Here's how the part is built. I have some questions about the finished solid (model axes, mm). Round coordinates to 2 decimals unless told otherwise and drop trailing zeros. Loops run counter-clockwise (first coordinate to the right, second up) from the corner with the lowest first, then second, coordinate; pieces in that order, holes last. Notation, with made-up numbers: (11, 75) - (58, 75) arc R18 cw to (58, 93) - close; hole circle Ø11 at (43, 5). An arc over 180 degrees is marked (long way). Answer as a JSON object with one key per item and string values. Group by question number.
1) Will these pins go through, and if not, where does the flat tip stop? P1, Ø6, axis at y = 5.5, z = 93.5, coming from the -X side; P2, Ø13, axis at x = 12, z = 63.5, coming from the +Y side; P3, Ø9.5, axis at y = 489.5, z = 82.5, coming from the +X side.
2) If I drill on line 1 along X through (y, z) = (73, 13.5), over which ranges is the centre line in solid material (lowest first)? Write a range as [from, to].
3) I want a section at C-C, the plane z = 46.5. Please give me the cut outline in (x, y), then the cut area to 3 significant figures.
4) I want a section at A-A, the plane y = 259.5. Please give me the cut outline in (x, z).
5) I want a section at B-B, the plane x = 310. Please give me the cut outline in (y, z).
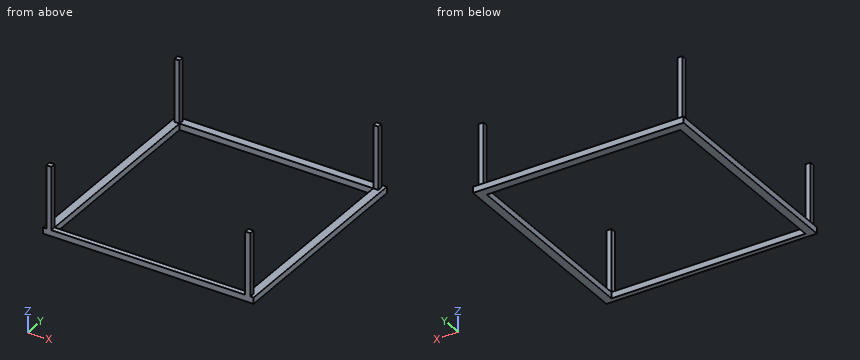
from build123d import *

# Parameters (mm, degrees)
SKETCH1_W           = 503
SKETCH1_H           = 503
SKETCH1_W_2         = 463
SKETCH1_H_2         = 471
BOSS_EXTRUDE1_DEPTH = 15
SKETCH2_W           = 12
SKETCH2_H           = 12
BOSS_EXTRUDE2_DEPTH = 200
SKETCH3_W           = 487
SKETCH3_H           = 495
CUT_EXTRUDE1_DEPTH  = 50


with BuildPart() as part:
    # Sketch1 → Boss-Extrude1 (new body)
    with BuildSketch(Plane.XY):
        with Locations((251.5, 251.5)):
            Rectangle(SKETCH1_W, SKETCH1_H)
        with Locations((251.5, 247.5)):
            Rectangle(SKETCH1_W_2, SKETCH1_H_2, mode=Mode.SUBTRACT)
    extrude(amount=BOSS_EXTRUDE1_DEPTH)

    # Sketch2 → Boss-Extrude2 (add)
    with BuildSketch(Plane.XY.offset(15)):
        with Locations((14, 489)):
            Rectangle(SKETCH2_W, SKETCH2_H)
        with Locations((489, 489)):
            Rectangle(SKETCH2_W, SKETCH2_H)
        with Locations((14, 6)):
            Rectangle(SKETCH2_W, SKETCH2_H)
        with Locations((489, 6)):
            Rectangle(SKETCH2_W, SKETCH2_H)
    extrude(amount=BOSS_EXTRUDE2_DEPTH)

    # Sketch3 → Cut-Extrude1 (cut)
    with BuildSketch(Plane.XY.offset(215)):
        with Locations((251.5, 247.5)):
            Rectangle(SKETCH3_W, SKETCH3_H)
    extrude(amount=-CUT_EXTRUDE1_DEPTH, mode=Mode.SUBTRACT)


solid = part.part
Outcome:
{
 "1": {"P1": "x = 8", "P2": "y = 495", "P3": "x = 495"},
 "2": {"line 1": "[0, 20], [483, 503]"},
 "3": {"outline": "(8, 0) - (20, 0) - (20, 12) - (8, 12) - close; (8, 483) - (20, 483) - (20, 495) - (8, 495) - close; (483, 0) - (495, 0) - (495, 12) - (483, 12) - close; (483, 483) - (495, 483) - (495, 495) - (483, 495) - close", "area": "576 mm^2"},
 "4": {"outline": "(0, 0) - (20, 0) - (20, 15) - (0, 15) - close; (483, 0) - (503, 0) - (503, 15) - (483, 15) - close"},
 "5": {"outline": "(0, 0) - (12, 0) - (12, 15) - (0, 15) - close; (483, 0) - (503, 0) - (503, 15) - (483, 15) - close"}
}
